For this review, take the finished solid that the model builds, in its own axes (mm). Face numbers are marked on the shaded views. Round coordinates to 2 decimals unless told otherwise and drop trailing zeros. Write each loop counter-clockwise with the first axis right and the second up, starting at its lowest first coordinate (ties: lowest second). Pieces come first, ordered by that corner, then holes.
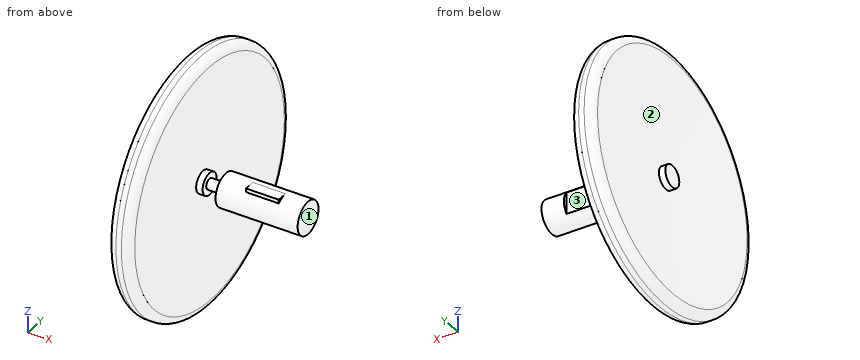
from build123d import *

# Parameters (mm, degrees)
SKETCH001_W  = 5.969217
SKETCH001_H  = 0.730541
POCKET_DEPTH = 33.001
SKETCH002_W  = 5.969217
SKETCH002_H  = 0.683974
PAD_DEPTH    = 2


with BuildPart() as part:
    # Sketch → Revolution (revolve)
    with BuildSketch(Plane.XY):
        with BuildLine():
            Line((1.5, 23), (2.5, 23))
            ThreePointArc((4, 21.5), (3.5606601718, 22.5606601718), (2.5, 23))
            Line((2.820253, 2), (4, 21.5))
            Line((4, 2), (2.820253, 2))
            Line((4, 0.960387), (4, 2))
            Line((4, 0.960387), (7, 0.960387))
            Line((7, 0.960387), (7, 3))
            Line((7, 3), (22, 3))
            Line((22, 3), (22, 0))
            Line((22, 0), (0, 0))
            Line((0, 0), (0, 2))
            Line((0, 2), (1.179747, 2))
            Line((1.179747, 2), (0, 21.5))
            ThreePointArc((1.5, 23), (0.4393398282, 22.5606601718), (0, 21.5))
        make_face()
    revolve(axis=Axis((0, 0, 0), (1, 0, 0)))

    # Sketch001 → Pocket (cut, through all)
    with BuildSketch(Plane.XY.offset(10)):
        with Locations((14.9151665, 2.6347295)):
            Rectangle(SKETCH001_W, SKETCH001_H)
    extrude(amount=-POCKET_DEPTH, mode=Mode.SUBTRACT)

    # Sketch002 → Pad (join)
    with BuildSketch(Plane.XZ):
        with Locations((14.9151665, 2.658013)):
            Rectangle(SKETCH002_W, SKETCH002_H)
    extrude(amount=PAD_DEPTH)


solid = part.part
(1) We need section B-B, the plane x = 5. Give the boundary of the cut face in (y, z), and give its area (3 significant figures).
Geometry check:
outline: circle Ø1.92 at (0, 0)
area: 2.90 mm2
(2) We need section C-C, the plane x = 10.75. Give the boundary of the cut face in (y, z).
Geometry check:
outline: circle Ø6 at (0, 0)
(3) For pin 1 Ø4 at (x, z) = (18.5, -5.5) entering from +Y; pin 2 Ø12 at (y, z) = (18, -9.5) entering from +X; pin 3 Ø1 at (y, z) = (-3, -14.5) entering from -X; pin 4 Ø4 at (x, z) = (2, -8.5) entering from +Y, all flat-tipped, find the tip position at first contact; note any pin that passes through.
Geometry check:
pin 1: passes through
pin 2: stops at x = 4
pin 3: stops at x = 0.37
pin 4: stops at y = 22.06
(4) We need section A-A, the plane z = 0. Give the boundary of the cut face in (x, y).
Geometry check:
outline: (0, -21.5) arc R1.5 ccw to (1.5, -23) - (2.5, -23) arc R1.5 ccw to (4, -21.5) - (2.82, -2) - (4, -2) - (4, -0.96) - (7, -0.96) - (7, -3) - (22, -3) - (22, 3) - (17.9, 3) - (17.9, 2.27) - (11.93, 2.27) - (11.93, 3) - (7, 3) - (7, 0.96) - (4, 0.96) - (4, 2) - (2.82, 2) - (4, 21.5) arc R1.5 ccw to (2.5, 23) - (1.5, 23) arc R1.5 ccw to (0, 21.5) - (1.18, 2) - (0, 2) - (0, -2) - (1.18, -2) - close
(5) For line 1 along X through (y, z) = (7.5, 2); line 2 along X through (y, z) = (9, -10.5); line 3 along Z through (x, y) = (1.75, -10.5), list the stretches that pass through material, from the lowest coordinate up.
Geometry check:
line 1: x = 0.83 to 3.17
line 2: x = 0.46 to 3.54
line 3: z = -20.46 to 20.46
(6) Mouldability with a two-part tool opening along X and no side actions: class the marked faces 1, 2 and 3 as pulls with the +X half, pulls with the -X half, needs draft (parallel to the pull), parting line crosses it, or undercut.
Geometry check:
face 1: pulls with the +X half
face 2: pulls with the -X half
face 3: undercut
